Model file for the job. Use its own axes, mm. Coordinates: 2 decimals unless noted, no trailing zeros. Loops run counter-clockwise (first coordinate to the right, second up) from the corner with the lowest first, then second, coordinate; pieces in that order, holes last. Notation, with made-up numbers: (-21.75, -1.5) - (36.25, -1.5) arc R14 ccw to (36.25, 24.5) - close; hole circle Ø11 at (-30, 43.25). An arc over 180 degrees is marked (long way). Write each question's results on one line, items separated by ' | '. Start each with the question number.
```python
from build123d import *

# Parameters (mm, degrees)
BOSS_EXTRUDE1_DEPTH = 3
SKETCH2_W           = 47
SKETCH2_H           = 8
CUT_EXTRUDE1_DEPTH  = 10


with BuildPart() as part:
    # Sketch1 → Boss-Extrude1 (new body)
    with BuildSketch(Plane.XZ.offset(548.298939869)):
        Polygon((-175.210843614, 789.620141885), (-47.210843614, 789.620141885), (-47.210843614, 389.620141885), (-60.218241118, 389.620141885), (-60.218241118, 474.220141885), (-98.410843614, 474.220141885), (-98.410843614, 449.620141885), (-124.010843614, 449.620141885), (-124.010843614, 474.220141885), (-161.818241118, 474.220141885), (-161.818241118, 389.620141885), (-175.210843614, 389.620141885), align=None)
    extrude(amount=BOSS_EXTRUDE1_DEPTH)

    # Sketch2 → Cut-Extrude1 (cut)
    with BuildSketch(Plane(origin=(0, -548.298939869, 0), x_dir=(1, 0, 0), z_dir=(0, 1, 0))):
        with Locations((-111.210843614, -789.620141885)):
            Rectangle(SKETCH2_W, SKETCH2_H)
    extrude(amount=-CUT_EXTRUDE1_DEPTH, mode=Mode.SUBTRACT)


solid = part.part
```
Q1. Pin check, flat tips, straight feed: pin 1 (1 mm diameter, centred on x = -128, y = -549.5, fed in from +Z); pin 2 (0.9 mm diameter, centred on x = -115.5, y = -550.5, fed in from -Z); pin 3 (0.9 mm diameter, centred on x = -70.5, y = -550.5, fed in from -Z). Stop position of each tip, or through.
Q2. Cut at C-C (x = -128). List the corners of the cut face in (y, z), and give its area (3 significant figures).
Q3. Cut at A-A (z = 454). List the corners of the cut face in (x, y).
Q4. Cut at D-D (x = -80). List the corners of the cut face in (y, z), and give its area (3 significant figures).
Q5. Cut at B-B (y = -550.3). List the corners of the cut face in (x, z), and give its area (3 significant figures).
Q6. Drill centre lines: L1, parallel to X at y = -549.55, z = 473.5; L2, parallel to X at y = -549.3, z = 417; L3, parallel to Z at x = -97, y = -548.8. Where is each one in solid material? Low to high. Write a range as from..to.
Check result:
1) pin 1: z = 785.62 | pin 2: z = 449.62 | pin 3: z = 474.22
2) outline: (-551.3, 474.22) - (-548.3, 474.22) - (-548.3, 785.62) - (-551.3, 785.62) - close | area: 934 mm²
3) outline: (-175.21, -551.3) - (-161.82, -551.3) - (-161.82, -548.3) - (-175.21, -548.3) - close; (-124.01, -551.3) - (-98.41, -551.3) - (-98.41, -548.3) - (-124.01, -548.3) - close; (-60.22, -551.3) - (-47.21, -551.3) - (-47.21, -548.3) - (-60.22, -548.3) - close
4) outline: (-551.3, 474.22) - (-548.3, 474.22) - (-548.3, 789.62) - (-551.3, 789.62) - close | area: 946 mm²
5) outline: (-175.21, 389.62) - (-161.82, 389.62) - (-161.82, 474.22) - (-124.01, 474.22) - (-124.01, 449.62) - (-98.41, 449.62) - (-98.41, 474.22) - (-60.22, 474.22) - (-60.22, 389.62) - (-47.21, 389.62) - (-47.21, 789.62) - (-87.71, 789.62) - (-87.71, 785.62) - (-134.71, 785.62) - (-134.71, 789.62) - (-175.21, 789.62) - close | area: 43,000 mm²
6) L1: -175.21..-161.82, -124.01..-98.41, -60.22..-47.21 | L2: -175.21..-161.82, -60.22..-47.21 | L3: 474.22..785.62
